from build123d import *

# Parameters (mm, degrees)
F1_DEPTH = 63.5
F3_W     = 50.8
F3_H     = 12.7
F4_DEPTH = 660.4
F2_W     = 12.7
F2_H     = 50.8
F5_DEPTH = 641.35
F6_W     = 63.5
F6_H     = 660.4
F7_DEPTH = 6.35


with BuildPart() as f1:
    # F0 (on Right) → F1 (new body)
    with BuildSketch(Plane.YZ):
        Polygon((-660.4, 0), (0, 0), (0, 38.1), (-177.8, 38.1), (-177.8, 19.05), (-482.6, 19.05), (-482.6, 38.1), (-660.4, 38.1), align=None)
    extrude(amount=F1_DEPTH)

    # F3 (on face) → F4 (join)
    with BuildSketch(Plane.XY.offset(19.05)):
        with Locations((31.75, -336.55)):
            Rectangle(F3_W, F3_H)
    extrude(amount=F4_DEPTH)

    # F2 (on face) → F5 (join)
    with BuildSketch(Plane.XY.offset(38.1)):
        with Locations((31.75, -571.5)):
            Rectangle(F2_W, F2_H)
        with Locations((31.75, -88.9)):
            Rectangle(F2_W, F2_H)
    extrude(amount=F5_DEPTH)

    # F6 (on face) → F7 (join)
    with BuildSketch(Plane.XY.offset(679.45)):
        with Locations((31.75, -330.2)):
            Rectangle(F6_W, F6_H)
    extrude(amount=F7_DEPTH)


solid = f1.part
Design review of the part built by this model. Coordinates are the model's own, in mm. A direction names the side the tool comes from. Give positions to 0.01 mm unless a question says otherwise; leave off trailing zeros. Order: outer loops, then holes, each group sorted by start corner. A loop starts at its lowest first (then second) coordinate and runs counter-clockwise, first axis right, second up. Notation, with made-up numbers: (87.5, 15) - (127.5, 15) arc R26 ccw to (127.5, 52) - close; hole circle Ø8 at (2.25, 53.5). An arc over 180 degrees is marked (long way). Write item = value, one per line. Start each with the question number.
Q1. We need section B-B on z = 337. State the section outline as (x, y) points.
Q2. Clearance check with flat-ended pins moving along their axes: pin 1 Ø10 at (y, z) = (-338.5, 93.5) entering from +X; pin 2 Ø4 at (x, z) = (32.5, 504.5) entering from +Y; pin 3 Ø10 at (x, z) = (6.5, 530.5) entering from -Y; pin 4 Ø10 at (x, y) = (38, -295.5) entering from -Z. State where each tip first meets the part, or that it passes through.
Q3. Tool access review of faces 5 (the face through (25.4, -89, 354)), 6 (the face through (31, -482.6, 28)), 7 (the face through (38.1, -89, 354)): name each direction out of +Z, -Z, +X, -X, +Y, -Y from which nothing blocks a thin tool from reaching the whole face with its end or side.
Q4. We need section A-A on y = -535. State the section outline as (x, z) points, plus the area to 3 significant figures.
Q5. We need section C-C on y = -224. State the section outline as (x, z) points, plus the area to 3 significant figures.
Q6. To check wall thickness, follow L1, parallel to Y at x = 30.5, z = 588; L2, parallel to Y at x = 30.5, z = 31; L3, parallel to Z at x = 29, y = -281.5. State the ranges of each line that lie inside material, in increasing order. Write a range as from..to.
Q7. Mouldability with a two-part tool opening along Y and no side actions: class faces 1 (the face through (38.1, -572, 354)), 2 (the face through (31, -660.4, 19)), 3 (the face through (31, 0, 19)), 4 (the face through (31, -342.9, 345)) as released by +Y, released by -Y, zero draft, split by the parting line, or undercut.
Working result:
q1.outline = (6.35, -342.9) - (57.15, -342.9) - (57.15, -330.2) - (6.35, -330.2) - close; (25.4, -596.9) - (38.1, -596.9) - (38.1, -546.1) - (25.4, -546.1) - close; (25.4, -114.3) - (38.1, -114.3) - (38.1, -63.5) - (25.4, -63.5) - close
q2.pin_1 = 57.15
q2.pin_2 = -63.5
q2.pin_3 = -342.9
q2.pin_4 = 0
q3.face_5 = -X, +Y
q3.face_6 = +X, -X
q3.face_7 = +X, +Y
q4.outline = (0, 0) - (63.5, 0) - (63.5, 38.1) - (0, 38.1) - close; (0, 679.45) - (63.5, 679.45) - (63.5, 685.8) - (0, 685.8) - close
q4.area = 2,820 mm²
q5.outline = (0, 0) - (63.5, 0) - (63.5, 19.05) - (0, 19.05) - close; (0, 679.45) - (63.5, 679.45) - (63.5, 685.8) - (0, 685.8) - close
q5.area = 1,610 mm²
q6.L1 = -596.9..-546.1, -342.9..-330.2, -114.3..-63.5
q6.L2 = -660.4..-482.6, -342.9..-330.2, -177.8..0
q6.L3 = 0..19.05, 679.45..685.8
q7.face_1 = zero draft
q7.face_2 = released by -Y
q7.face_3 = released by +Y
q7.face_4 = undercut
